from build123d import *

# Parameters (mm, degrees)
SKETCH1_W                   = 54
SKETCH1_H                   = 65
BOSS_EXTRUDE1_DEPTH         = 50
SKETCH2_W                   = 21
SKETCH2_H                   = 41.5
CUT_EXTRUDE1_DEPTH          = 99.188594042
FILLET1_R                   = 6
SKETCH3_W                   = 21
SKETCH3_H                   = 56
CUT_EXTRUDE2_DEPTH          = 42
CUT_EXTRUDE_THIN3_DEPTH     = 15.67
CUT_EXTRUDE3_DEPTH          = 15.67
M5_TAPPED_HOLE1_D           = 4.2
M5_TAPPED_HOLE1_DEPTH       = 15
M5_TAPPED_HOLE1_CSINK_D     = 5.05
M5_TAPPED_HOLE1_CSINK_ANGLE = 90
M5_TAPPED_HOLE1_TIP         = 1.2618073
M3_TAPPED_HOLE1_D           = 2.5
M3_TAPPED_HOLE1_CSINK_D     = 3.05
M3_TAPPED_HOLE1_CSINK_ANGLE = 90
HOLE1_D                     = 6.5
HOLE1_CBORE_D               = 11
HOLE1_CBORE_DEPTH           = 7
EXTRUDE_THIN1_START         = 1.5
EXTRUDE_THIN1_DEPTH         = 1.5
M3_TAPPED_HOLE2_D           = 2.5
M3_TAPPED_HOLE2_CSINK_D     = 3.05
M3_TAPPED_HOLE2_CSINK_ANGLE = 90


with BuildPart() as part:
    # Sketch1 → Boss-Extrude1 (new body)
    with BuildSketch(Plane.XY):
        with Locations((27, 32.5)):
            Rectangle(SKETCH1_W, SKETCH1_H)
    extrude(amount=BOSS_EXTRUDE1_DEPTH)

    # Sketch2 → Cut-Extrude1 (cut, through all)
    with BuildSketch(Plane.XY.offset(50)):
        with Locations((27, 32.5)):
            Rectangle(SKETCH2_W, SKETCH2_H)
    extrude(amount=-CUT_EXTRUDE1_DEPTH, mode=Mode.SUBTRACT)

    # Fillet1
    fillet1_edges = [part.edges().sort_by_distance(p)[0] for p in [
        (0, 65, 25),
        (54, 65, 25),
        (54, 0, 25),
        (0, 0, 25),
    ]]
    fillet(fillet1_edges, radius=FILLET1_R)

    # Sketch3 → Cut-Extrude2 (cut)
    with BuildSketch(Plane.XY.offset(50)):
        with Locations((27, 32.5)):
            Rectangle(SKETCH3_W, SKETCH3_H)
    extrude(amount=-CUT_EXTRUDE2_DEPTH, mode=Mode.SUBTRACT)

    # Sketch4 → Cut-Extrude-Thin3 (cut)
    with BuildSketch(Plane.XY.offset(50)):
        with BuildLine():
            Line((6.119863014, 48.642808121), (20.863013699, 55.83321895))
            ThreePointArc((20.863013699, 55.83321895), (27, 57.25), (33.136986301, 55.83321895))
            Line((33.136986301, 55.83321895), (47.880136986, 48.642808121))
            ThreePointArc((47.880136986, 48.642808121), (51.25, 43.25), (47.880136986, 37.857191879))
            Line((47.880136986, 37.857191879), (33.136986301, 30.66678105))
            ThreePointArc((33.136986301, 30.66678105), (27, 29.25), (20.863013699, 30.66678105))
            Line((20.863013699, 30.66678105), (6.119863014, 37.857191879))
            ThreePointArc((6.119863014, 37.857191879), (2.75, 43.25), (6.119863014, 48.642808121))
        make_face()
        with BuildLine():
            Line((6.339041096, 48.193407445), (21.082191781, 55.383818273))
            ThreePointArc((21.082191781, 55.383818273), (27, 56.75), (32.917808219, 55.383818273))
            Line((32.917808219, 55.383818273), (47.660958904, 48.193407445))
            ThreePointArc((47.660958904, 48.193407445), (50.75, 43.25), (47.660958904, 38.306592555))
            Line((47.660958904, 38.306592555), (32.917808219, 31.116181727))
            ThreePointArc((32.917808219, 31.116181727), (27, 29.75), (21.082191781, 31.116181727))
            Line((21.082191781, 31.116181727), (6.339041096, 38.306592555))
            ThreePointArc((6.339041096, 38.306592555), (3.25, 43.25), (6.339041096, 48.193407445))
        make_face(mode=Mode.SUBTRACT)
    extrude(amount=-CUT_EXTRUDE_THIN3_DEPTH, mode=Mode.SUBTRACT)

    # Sketch4<3> → Cut-Extrude3 (cut)
    with BuildSketch(Plane.XY.offset(50)):
        with BuildLine():
            Line((32.917808219, 55.383818273), (47.660958904, 48.193407445))
            ThreePointArc((47.660958904, 48.193407445), (50.75, 43.25), (47.660958904, 38.306592555))
            Line((47.660958904, 38.306592555), (32.917808219, 31.116181727))
            ThreePointArc((32.917808219, 31.116181727), (27, 29.75), (21.082191781, 31.116181727))
            Line((21.082191781, 31.116181727), (6.339041096, 38.306592555))
            ThreePointArc((6.339041096, 38.306592555), (3.25, 43.25), (6.339041096, 48.193407445))
            Line((6.339041096, 48.193407445), (21.082191781, 55.383818273))
            ThreePointArc((21.082191781, 55.383818273), (27, 56.75), (32.917808219, 55.383818273))
        make_face()
    extrude(amount=-CUT_EXTRUDE3_DEPTH, mode=Mode.SUBTRACT)

    # M5 Tapped Hole1
    with Locations(Plane(origin=(8.75, 43.25, 34.33), x_dir=(1, 0, 0), z_dir=(0, 0, 1))):
        with Locations((0, 0), (36.5, 0)):
            CounterSinkHole(M5_TAPPED_HOLE1_D / 2, M5_TAPPED_HOLE1_CSINK_D / 2, depth=M5_TAPPED_HOLE1_DEPTH, counter_sink_angle=M5_TAPPED_HOLE1_CSINK_ANGLE)
            with Locations((0, 0, -(M5_TAPPED_HOLE1_DEPTH + M5_TAPPED_HOLE1_TIP / 2))):  # 118° drill point
                Cone(0, M5_TAPPED_HOLE1_D / 2, M5_TAPPED_HOLE1_TIP, mode=Mode.SUBTRACT)

    # M3 Tapped Hole1 (through all)
    with Locations(Plane(origin=(22, 56.85, 8), x_dir=(1, 0, 0), z_dir=(0, 0, 1))):
        with Locations((0, 0), (10, 0), (10, -48.7), (0, -48.7)):
            CounterSinkHole(M3_TAPPED_HOLE1_D / 2, M3_TAPPED_HOLE1_CSINK_D / 2, counter_sink_angle=M3_TAPPED_HOLE1_CSINK_ANGLE)

    # Hole1 (through all)
    with Locations(Plane(origin=(8.25, 56.75, 50), x_dir=(1, 0, 0), z_dir=(0, 0, 1))):
        with Locations((0, 0), (37.5, 0), (37.5, -48.5), (0, -48.5)):
            CounterBoreHole(HOLE1_D / 2, HOLE1_CBORE_D / 2, HOLE1_CBORE_DEPTH)

    # Sketch10 → Extrude-Thin1 (add)
    with BuildSketch(Plane.XY.offset(50).offset(EXTRUDE_THIN1_START)):
        with BuildLine():
            Line((48, 65), (6, 65))
            ThreePointArc((6, 65), (1.757359313, 63.242640687), (0, 59))
            Line((0, 59), (0, 6))
            ThreePointArc((0, 6), (1.757359313, 1.757359313), (6, 0))
            Line((6, 0), (48, 0))
            ThreePointArc((48, 0), (52.242640687, 1.757359313), (54, 6))
            Line((54, 6), (54, 59))
            ThreePointArc((54, 59), (52.242640687, 63.242640687), (48, 65))
        make_face()
        with BuildLine():
            Line((48, 63.5), (6, 63.5))
            ThreePointArc((6, 63.5), (2.818019485, 62.181980515), (1.5, 59))
            Line((1.5, 59), (1.5, 6))
            ThreePointArc((1.5, 6), (2.818019485, 2.818019485), (6, 1.5))
            Line((6, 1.5), (48, 1.5))
            ThreePointArc((48, 1.5), (51.181980515, 2.818019485), (52.5, 6))
            Line((52.5, 6), (52.5, 59))
            ThreePointArc((52.5, 59), (51.181980515, 62.181980515), (48, 63.5))
        make_face(mode=Mode.SUBTRACT)
    extrude(amount=-EXTRUDE_THIN1_DEPTH)

    # M3 Tapped Hole2 (through all)
    with Locations(Plane(origin=(8.25, 24.550881691, 50), x_dir=(1, 0, 0), z_dir=(0, 0, 1))):
        with Locations((0, 0), (37.5, 0)):
            CounterSinkHole(M3_TAPPED_HOLE2_D / 2, M3_TAPPED_HOLE2_CSINK_D / 2, counter_sink_angle=M3_TAPPED_HOLE2_CSINK_ANGLE)


solid = part.part
Build history of the part. All positions in model axes, mm. A direction names the side the tool comes from. Round coordinates to 2 decimals unless told otherwise and drop trailing zeros. Write each loop counter-clockwise with the first axis right and the second up, starting at its lowest first coordinate (ties: lowest second). Pieces come first, ordered by that corner, then holes. Notation, with made-up numbers: (12, 46.5) - (31, 46.5) arc R13 ccw to (31, 58.5) - close; hole circle Ø7 at (-6, -10). An arc over 180 degrees is marked (long way). Use CSV: the item, a comma, the result in double quotes.
(1) 3-axis set-ups, long thin cutter, end or side, ignore diameter. For faces 4 (the flat face through (48, 54, 43)), 5 (the flat face through (27, 53.25, 4)): which of +Z, -Z, +X, -X, +Y, -Y reach the whole face in a straight line?
Response:
face 4,"+Z"
face 5,"+Z, -Z"
(2) Pin check, flat tips, straight feed: P1, Ø4, axis at x = 36, y = 22.5, coming from the +Z side; P2, Ø4, axis at x = 8.75, y = 43.25, coming from the +Z side; P3, Ø7.5, axis at x = 8.25, y = 8.25, coming from the +Z side. Stop position of each tip, or through.
Response:
P1,"z = 50"
P2,"z = 19.27"
P3,"z = 43"
(3) Wall check: line 1 (Y direction, x = 32, z = 3); line 2 (X direction, y = 8, z = 45); line 3 (X direction, y = 30, z = 14.5). Give the ranges that are in metal, low to high.
Response:
line 1,"0 to 6.9, 9.4 to 11.75, 53.25 to 55.6, 58.1 to 65"
line 2,"0 to 2.76, 13.74 to 16.5, 37.5 to 40.26, 51.24 to 54"
line 3,"0 to 16.5, 37.5 to 54"
(4) Band-saw the part on B-B (z = 37). Write the cut outline in (x, y), plus the area to 3 significant figures.
Response:
outline,"(0, 6) arc R6 ccw to (6, 0) - (48, 0) arc R6 ccw to (54, 6) - (54, 59) arc R6 ccw to (48, 65) - (6, 65) arc R6 ccw to (0, 59) - close; hole circle Ø6.5 at (8.25, 8.25); hole circle Ø6.5 at (8.25, 56.75); hole (6.12, 37.86) - (16.5, 32.79) - (16.5, 4.5) - (37.5, 4.5) - (37.5, 32.79) - (47.88, 37.86) arc R6 ccw to (47.88, 48.64) - (37.5, 53.71) - (37.5, 60.5) - (16.5, 60.5) - (16.5, 53.71) - (6.12, 48.64) arc R6 ccw to start; hole circle Ø2.5 at (8.25, 24.55); hole circle Ø6.5 at (45.75, 8.25); hole circle Ø6.5 at (45.75, 56.75); hole circle Ø2.5 at (45.75, 24.55)"
area,"1,780 mm²"
(5) Band-saw the part on C-C (z = 9). Write the cut outline in (x, y), plus the area to 3 significant figures.
Response:
outline,"(0, 6) arc R6 ccw to (6, 0) - (48, 0) arc R6 ccw to (54, 6) - (54, 59) arc R6 ccw to (48, 65) - (6, 65) arc R6 ccw to (0, 59) - close; hole circle Ø6.5 at (8.25, 8.25); hole circle Ø6.5 at (8.25, 56.75); hole circle Ø2.5 at (8.25, 24.55); hole (16.5, 4.5) - (37.5, 4.5) - (37.5, 60.5) - (16.5, 60.5) - close; hole circle Ø6.5 at (45.75, 8.25); hole circle Ø6.5 at (45.75, 56.75); hole circle Ø2.5 at (45.75, 24.55)"
area,"2,160 mm²"
(6) Band-saw the part on A-A (x = 18). Write the cut outline in (y, z).
Response:
outline,"(0, 0) - (11.75, 0) - (11.75, 8) - (4.5, 8) - (4.5, 50) - (1.5, 50) - (1.5, 51.5) - (0, 51.5) - close; (53.25, 0) - (65, 0) - (65, 51.5) - (63.5, 51.5) - (63.5, 50) - (60.5, 50) - (60.5, 8) - (53.25, 8) - close"
(7) Mould opens along Y. For faces 1 (the flat face through (27, 0, 26)), 2 (the flat face through (1, 35, 51.5)), 3 (the cylindrical face through (51.217, 62.147, 50.76)) say: pulls with the +Y half, pulls with the -Y half, needs draft (parallel to the pull), parting line crosses it, or undercut.
Response:
face 1,"pulls with the -Y half"
face 2,"needs draft"
face 3,"undercut"
